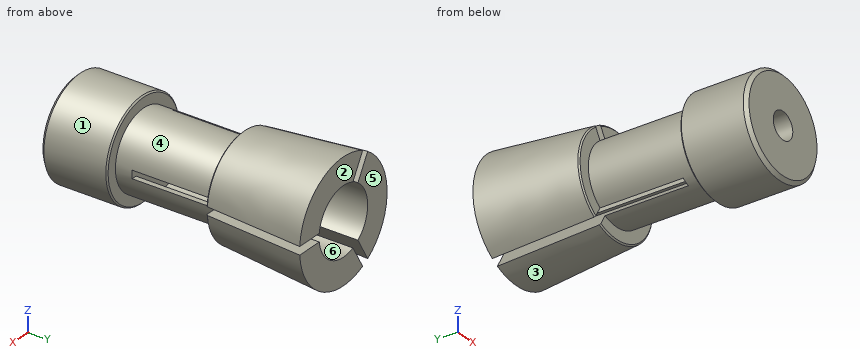
```python
from build123d import *

# Parameters (mm, degrees)
F2_R         = 6.35
F3_DEPTH     = 34.925
F5_D         = 5.1054
F9_DEPTH     = 34.925
F10_SIZE     = 0.635
F11_T4_ANGLE = 118.0970990721
F11_T6_ANGLE = 118.1103265481
F11_T8_ANGLE = 118.1037128101


# Not quite as in the source:
# - a fillet or chamfer that OpenCascade refuses, or shapes differently, is made with other operations: its cross-section is extruded or revolved along the edge and cut away or added


with BuildPart() as f1:
    # F0 (on Right) → F1 (revolve)
    with BuildSketch(Plane.YZ):
        Polygon((-11.3264165741, 23.7704595025), (-40.3521669373, 23.7704595025), (-40.3521669373, 14.2454595025), (10.4478330627, 14.2454595025), (10.4478330627, 25.6754595025), align=None)
    revolve(axis=Axis((0, -14.9521669373, 14.2454595025), (0, 1, 0)))

    # F2 (on face) → F3 (cut)
    with BuildSketch(Plane(origin=(0, 10.4478330627, 0), x_dir=(-1, 0, 0), z_dir=(0, 1, 0))):
        with Locations((0, 14.2454595025)):
            Circle(F2_R)
    extrude(amount=-F3_DEPTH, mode=Mode.SUBTRACT)

    # F5 (through all)
    with Locations(Plane.XZ.offset(40.3521669373)):
        with Locations((0, 14.2454595025)):
            Hole(F5_D / 2)

    # F6 (on Right) → F7 (revolve, cut)
    with BuildSketch(Plane.YZ):
        Polygon((-11.3264165741, 23.7704595025), (-27.6521669373, 23.7704595025), (-27.6521669373, 21.6114595025), (-8.6021669373, 21.6114595025), (-8.6021669373, 24.0088004624), align=None)
    revolve(axis=Axis((0, -14.9521669373, 14.2454595025), (0, 1, 0)), mode=Mode.SUBTRACT)

    # F8 (on face) → F9 (cut)
    with BuildSketch(Plane(origin=(0, 10.4478330627, 0), x_dir=(-1, 0, 0), z_dir=(0, 1, 0))):
        with BuildLine():
            Line((-6.3041142122, 15.0074595025), (-11.4045717149, 15.0074595025))
            ThreePointArc((-11.4045717149, 15.0074595025), (-11.43, 14.2454595025), (-11.4045717149, 13.4834595025))
            Line((-11.4045717149, 13.4834595025), (-6.3041142122, 13.4834595025))
            ThreePointArc((-6.3041142122, 13.4834595025), (-6.35, 14.2454595025), (-6.3041142122, 15.0074595025))
        make_face()
        with BuildLine():
            Line((3.8113822624, 19.3244225118), (6.3611011609, 23.7418426046))
            ThreePointArc((6.3611011609, 23.7418426046), (5.7138574323, 24.1447894416), (5.0411905024, 24.5036902622))
            Line((5.0411905024, 24.5036902622), (2.4914716038, 20.0862701695))
            ThreePointArc((2.4914716038, 20.0862701695), (3.1743652402, 19.7450872465), (3.8113822624, 19.3244225118))
        make_face()
        with BuildLine():
            ThreePointArc((5.04355843, 3.9883927501), (5.7161424915, 4.347448843), (6.3632931846, 4.7505450823))
            Line((6.3632931846, 4.7505450823), (3.8125546144, 9.1673764673))
            ThreePointArc((3.8125546144, 9.1673764673), (3.1756347175, 8.7465646917), (2.4928198598, 8.4052241351))
            Line((2.4928198598, 8.4052241351), (5.04355843, 3.9883927501))
        make_face()
    extrude(amount=-F9_DEPTH, mode=Mode.SUBTRACT)

    # F10
    f10_edges = [f1.edges().sort_by_distance(p)[0] for p in [
        (0, -40.352167, 4.72046),
    ]]
    chamfer(f10_edges, length=F10_SIZE)

    # F11: chamfer of 0.254 on 4 edges, made by hand

    # F11_s1 → F11_t2 (revolve, cut)
    with BuildSketch(Plane.YZ):
        Polygon((-27.9061669373, 23.7704595025), (-27.6521669373, 23.5164595025), (-27.6521669373, 23.7704595025), align=None)
    revolve(axis=Axis((0, -27.6521669373, 14.2454595025), (0, 1, 0)), mode=Mode.SUBTRACT)

    # F11_s3 → F11_t4 (revolve, cut)
    with BuildSketch(Plane(origin=(6.0463708023, 0, 3.3578022312), x_dir=(0, 1, 0), z_dir=(-0.8742366104, 0, -0.485500102))):
        Polygon((-8.6021669373, -21.9844950709), (-8.3703044959, -22.2375285242), (-8.6021669373, -22.2172431891), align=None)
    revolve(axis=Axis((0, -8.6021669373, 14.2454595025), (0, 1, 0)), revolution_arc=F11_T4_ANGLE, mode=Mode.SUBTRACT)

    # F11_s5 → F11_t6 (revolve, cut)
    with BuildSketch(Plane(origin=(0.2356940066, 0, 14.2415588295), x_dir=(0, 1, 0), z_dir=(0.0165474678, 0, 0.9998630813))):
        Polygon((-8.6021669373, -9.2948665597), (-8.3703044959, -9.547900013), (-8.6021669373, -9.5276146779), align=None)
    revolve(axis=Axis((0, -8.6021669373, 14.2454595025), (0, 1, 0)), revolution_arc=F11_T6_ANGLE, mode=Mode.SUBTRACT)

    # F11_s7 → F11_t8 (revolve, cut)
    with BuildSketch(Plane(origin=(-6.2837082468, 0, 3.7688827395), x_dir=(0, 1, 0), z_dir=(0.8575737294, 0, -0.5143610587))):
        Polygon((-8.6021669373, 2.6859389904), (-8.3703044959, 2.4329055371), (-8.6021669373, 2.4531908722), align=None)
    revolve(axis=Axis((0, -8.6021669373, 14.2454595025), (0, 1, 0)), revolution_arc=F11_T8_ANGLE, mode=Mode.SUBTRACT)


solid = f1.part
```
The listing builds one solid part. Answer for the finished solid, in the listing's coordinates (mm). Face numbers are marked on the shaded views. A direction names the side the tool comes from. Round coordinates to 2 decimals unless told otherwise and drop trailing zeros. Write each loop counter-clockwise with the first axis right and the second up, starting at its lowest first coordinate (ties: lowest second). Pieces come first, ordered by that corner, then holes. Notation, with made-up numbers: (-38, 19.5) -> (11, 19.5) arc R22 cw to (11, 44.5) -> close; hole circle Ø3 at (17, 28). An arc over 180 degrees is marked (long way). Write item = value, one per line.
1) Section B-B on y = -1.5 is taken. Write down the section's boundary in (x, z).
Check values:
outline = (-5.84, 5.66) -> (-3.81, 9.17) arc R6.35 cw to (-3.81, 19.32) -> (-5.84, 22.83) arc R10.38 ccw to start; (-4.52, 4.9) arc R10.38 ccw to (10.36, 13.48) -> (6.3, 13.48) arc R6.35 cw to (-2.49, 8.41) -> close; (-4.52, 23.6) -> (-2.49, 20.09) arc R6.35 cw to (6.3, 15.01) -> (10.36, 15.01) arc R10.38 ccw to start
2) Which of the six approach directions +Z, -Z, +X, -X, +Y, -Y give full straight-line access (tool end or side, diameter ignored) to the marked faces 5 and 6?
Check values:
face_5 = +Z, -Z, +X, -X, +Y
face_6 = +Y
3) Straight lines are drawn through the part: line 1 along Y through (x, z) = (-8.25, 14); line 2 along Y through (x, z) = (-2.5, 13.25); line 3 along X through (y, z) = (-21, 19). For each, find the intervals that lie inside material, in ascending order. Write a range as [from, to].
Check values:
line_1 = [-40.35, -27.65], [-8.6, 10.45]
line_2 = [-40.35, -24.48]
line_3 = [-5.63, -4.21], [4.21, 5.63]
4) Section A-A on x = 0 is taken. Write down the section's boundary in (y, z), plus the area to 3 significant figures.
Check values:
outline = (-40.35, 5.36) -> (-39.72, 4.72) -> (-27.91, 4.72) -> (-27.65, 4.97) -> (-27.65, 6.88) -> (-8.6, 6.88) -> (-8.6, 4.71) -> (-8.37, 4.46) -> (10.45, 2.82) -> (10.45, 7.9) -> (-24.48, 7.9) -> (-24.48, 11.69) -> (-40.35, 11.69) -> close; (-40.35, 16.8) -> (-24.48, 16.8) -> (-24.48, 20.6) -> (10.45, 20.6) -> (10.45, 25.68) -> (-8.37, 24.03) -> (-8.6, 23.78) -> (-8.6, 21.61) -> (-27.65, 21.61) -> (-27.65, 23.52) -> (-27.91, 23.77) -> (-39.72, 23.77) -> (-40.35, 23.14) -> close
area = 401 mm²
5) Given pin 1 (2 mm diameter, centred on x = -3, y = -29.5, fed in from +Z); pin 2 (3 mm diameter, centred on x = 2.5, y = -27.5, fed in from +Z); pin 3 (4 mm diameter, centred on x = 9, y = 1.5, fed in from -Z); pin 4 (6 mm diameter, centred on x = 0, z = 14.25, fed in from -Y), each flat-ended and moving along its own axis, determine where each tip first touches the part or whether it passes through.
Check values:
pin_1 = 23.56
pin_2 = 23.71
pin_3 = 6.21
pin_4 = -40.35
6) For a pull along Y with two mould halves and no side action, classify the marked faces 1, 2, 3 and 4 as released by +Y, released by -Y, zero draft, split by the parting line, or undercut.
Check values:
face_1 = zero draft
face_2 = released by +Y
face_3 = released by -Y
face_4 = undercut
7) Section C-C on y = -21.5 is taken. Write down the section's boundary in (x, z), plus the area to 3 significant figures.
Check values:
outline = (-4.32, 8.28) -> (-3.81, 9.17) arc R6.35 cw to (-3.81, 19.32) -> (-4.32, 20.21) arc R7.37 ccw to start; (-3, 7.52) arc R7.37 ccw to (7.33, 13.48) -> (6.3, 13.48) arc R6.35 cw to (-2.49, 8.41) -> close; (-3, 20.97) -> (-2.49, 20.09) arc R6.35 cw to (6.3, 15.01) -> (7.33, 15.01) arc R7.37 ccw to start
area = 39.1 mm²
